The model under review builds one solid part; all positions refer to its coordinate system, in mm. Face numbers are marked on the shaded views. Round coordinates to 2 decimals unless told otherwise and drop trailing zeros. Write each loop counter-clockwise with the first axis right and the second up, starting at its lowest first coordinate (ties: lowest second). Pieces come first, ordered by that corner, then holes. Notation, with made-up numbers: (32, 63) -> (61, 63) arc R32 cw to (61, 95) -> close; hole circle Ø8 at (49, 23.5). An arc over 180 degrees is marked (long way). Answer in a Markdown table with one row per item. Add a question column.
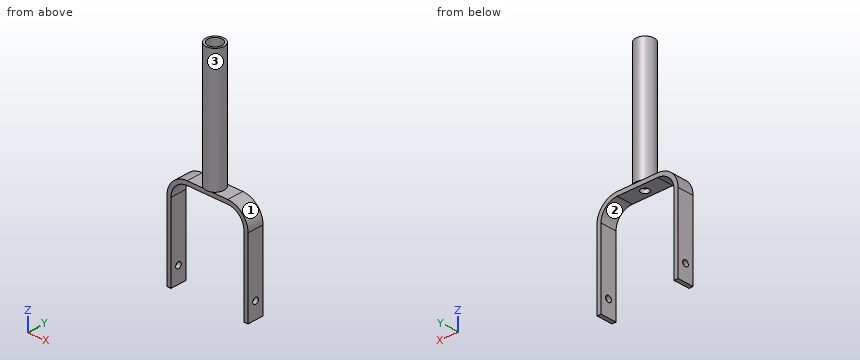
```python
from build123d import *

# Parameters (mm, degrees)
F1_DEPTH = 12.7
F2_R     = 25.4
F3_R     = 31.75
F5_D     = 9.525
F7_D     = 12.7
F8_R     = 14.2875
F8_R_2   = 11.1125
F9_DEPTH = 190.5


with BuildPart() as f1:
    # F0 (on Front) → F1 (new body, symmetric)
    with BuildSketch(Plane.XZ):
        Polygon((0, 152.4), (0, 0), (6.35, 0), (6.35, 146.05), (120.65, 146.05), (120.65, 0), (127, 0), (127, 152.4), align=None)
    extrude(amount=F1_DEPTH, both=True)

    # F2
    f2_edges = [f1.edges().sort_by_distance(p)[0] for p in [
        (6.35, 0, 146.05),
        (120.65, 0, 146.05),
    ]]
    fillet(f2_edges, radius=F2_R)

    # F3
    f3_edges = [f1.edges().sort_by_distance(p)[0] for p in [
        (127, 0, 152.4),
        (0, 0, 152.4),
    ]]
    fillet(f3_edges, radius=F3_R)

    # F5 (through all)
    with Locations(Plane(origin=(0, 0, 0), x_dir=(0, 1, 0), z_dir=(-1, 0, 0))):
        with Locations((0, -25.4)):
            Hole(F5_D / 2)

    # F7 (through all)
    with Locations(Plane.XY.offset(152.4)):
        with Locations((63.5, 0)):
            Hole(F7_D / 2)

    # F8 (on face) → F9 (join)
    with BuildSketch(Plane.XY.offset(152.4)):
        with Locations((63.5, 0)):
            Circle(F8_R)
        with Locations((63.5, 0)):
            Circle(F8_R_2, mode=Mode.SUBTRACT)
    extrude(amount=F9_DEPTH)


solid = f1.part
```
1. Add section D-D on x = 87.5. Write out the cut boundary in (y, z).
2. Insertion check: pin 1 Ø1 at (x, y) = (108, -2.5) entering from -Z; pin 2 Ø11 at (y, z) = (0, 25.4) entering from -X; pin 3 Ø1 at (x, y) = (22.5, -8) entering from -Z; pin 4 Ø4 at (x, y) = (111, -2) entering from -Z. Each pin has a flat end and moves straight along its axis. Give the tip position at first contact, or say it passes through.
3. Mouldability with a two-part tool opening along X and no side actions: class the marked faces 1, 2 and 3 as pulls with the +X half, pulls with the -X half, needs draft (parallel to the pull), parting line crosses it, or undercut.
4. Add section C-C on z = 239. Write out the cut boundary in (x, y) (1 decimal), plus the area to 3 significant figures.
5. Add section A-A on z = 48.5. Write out the cut boundary in (x, y), plus the area to 3 significant figures.
6. Add section B-B on x = 63.5. Write out the cut boundary in (y, z).
7. For L1, parallel to Y at x = 63.5, z = 149; L2, parallel to X at y = 1, z = 67; L3, parallel to X at y = 9, z = 323.5, list the stretches that pass through material, from the lowest coordinate up.
Filled in:
| question | item | result |
|---|---|---|
| 1 | outline | (-12.7, 146.05) -> (12.7, 146.05) -> (12.7, 152.4) -> (-12.7, 152.4) -> close |
| 2 | pin 1 | z = 142.32 |
| 2 | pin 2 | x = 0 |
| 2 | pin 3 | z = 144.1 |
| 2 | pin 4 | z = 138.82 |
| 3 | face 1 | pulls with the +X half |
| 3 | face 2 | undercut |
| 3 | face 3 | parting line crosses it |
| 4 | outline | circle Ø28.6 at (63.5, 0); hole circle Ø22.2 at (63.5, 0) |
| 4 | area | 253 mm² |
| 5 | outline | (0, -12.7) -> (6.35, -12.7) -> (6.35, 12.7) -> (0, 12.7) -> close; (120.65, -12.7) -> (127, -12.7) -> (127, 12.7) -> (120.65, 12.7) -> close |
| 5 | area | 323 mm² |
| 6 | outline | (-14.29, 152.4) -> (-12.7, 152.4) -> (-12.7, 146.05) -> (-6.35, 146.05) -> (-6.35, 152.4) -> (-11.11, 152.4) -> (-11.11, 342.9) -> (-14.29, 342.9) -> close; (6.35, 146.05) -> (12.7, 146.05) -> (12.7, 152.4) -> (14.29, 152.4) -> (14.29, 342.9) -> (11.11, 342.9) -> (11.11, 152.4) -> (6.35, 152.4) -> close |
| 7 | L1 | -12.7 to -6.35, 6.35 to 12.7 |
| 7 | L2 | 0 to 6.35, 120.65 to 127 |
| 7 | L3 | 52.4 to 56.98, 70.02 to 74.6 |
